Geometry check sheet. Reference: the model listing, model coordinates, mm. Coordinates: 2 decimals unless noted, no trailing zeros. Loops run counter-clockwise (first coordinate to the right, second up) from the corner with the lowest first, then second, coordinate; pieces in that order, holes last. Notation, with made-up numbers: (-35.5, 63) - (5.5, 63) arc R26 ccw to (5.5, 77) - close; hole circle Ø9 at (-36.75, 25). An arc over 180 degrees is marked (long way). One line per item, written item: value.
from build123d import *

# Parameters (mm, degrees)
SKETCH1_W           = 244
SKETCH1_H           = 158.15
BOSS_EXTRUDE1_DEPTH = 5
CUT_EXTRUDE1_DEPTH  = 10
SKETCH3_R           = 2.5
CUT_EXTRUDE2_DEPTH  = 10
SKETCH4_R           = 1
CUT_EXTRUDE3_DEPTH  = 10
SKETCH5_R           = 2
CUT_EXTRUDE4_DEPTH  = 10
CUT_EXTRUDE5_DEPTH  = 10


with BuildPart() as part:
    # Sketch1 → Boss-Extrude1 (new body)
    with BuildSketch(Plane.XY):
        with Locations((14.8, -10.925)):
            Rectangle(SKETCH1_W, SKETCH1_H)
    extrude(amount=BOSS_EXTRUDE1_DEPTH)

    # Sketch2 → Cut-Extrude1 (cut)
    with BuildSketch(Plane(origin=(0, 0, 0), x_dir=(-1, 0, 0), z_dir=(0, 0, -1))):
        Polygon((-136.8, 45.15), (-129.8, 45.15), (-129.8, 45.9), (-127.4, 45.9), (-127.4, 45.15), (-119.8, 45.15), (-119.8, 41.15), (-127.4, 41.15), (-127.4, 40.4), (-129.8, 40.4), (-129.8, 41.15), (-136.8, 41.15), align=None)
        Polygon((-129.8, -63), (-136.8, -63), (-136.8, -67), (-129.8, -67), (-129.8, -67.75), (-127.4, -67.75), (-127.4, -67), (-119.8, -67), (-119.8, -63), (-127.4, -63), (-127.4, -62.25), (-129.8, -62.25), align=None)
        Polygon((100.2, 41.15), (107.2, 41.15), (107.2, 45.15), (100.2, 45.15), (100.2, 45.9), (97.8, 45.9), (97.8, 45.15), (90.2, 45.15), (90.2, 41.15), (97.8, 41.15), (97.8, 40.4), (100.2, 40.4), align=None)
        Polygon((107.2, -67), (100.2, -67), (100.2, -67.75), (97.8, -67.75), (97.8, -67), (90.2, -67), (90.2, -63), (97.8, -63), (97.8, -62.25), (100.2, -62.25), (100.2, -63), (107.2, -63), align=None)
    extrude(amount=-CUT_EXTRUDE1_DEPTH, mode=Mode.SUBTRACT)

    # Sketch3 → Cut-Extrude2 (cut)
    with BuildSketch(Plane(origin=(0, 0, 0), x_dir=(-1, 0, 0), z_dir=(0, 0, -1))):
        with Locations((-124.8, -75.004567899)):
            Circle(SKETCH3_R)
        with Locations((-79.8, 48.15)):
            Circle(SKETCH3_R)
        with Locations((95.2, -75.004567899)):
            Circle(SKETCH3_R)
        with Locations((50.2, 48.15)):
            Circle(SKETCH3_R)
    extrude(amount=-CUT_EXTRUDE2_DEPTH, mode=Mode.SUBTRACT)

    # Sketch4 → Cut-Extrude3 (cut)
    with BuildSketch(Plane(origin=(0, 0, 0), x_dir=(-1, 0, 0), z_dir=(0, 0, -1))):
        with Locations((-38.8, 38.15)):
            Circle(SKETCH4_R)
        with Locations((1.2, 38.15)):
            Circle(SKETCH4_R)
        with Locations((-45.8, -32.925)):
            Circle(SKETCH4_R)
        with Locations((11.2, -32.925)):
            Circle(SKETCH4_R)
    extrude(amount=-CUT_EXTRUDE3_DEPTH, mode=Mode.SUBTRACT)

    # Sketch5 → Cut-Extrude4 (cut)
    with BuildSketch(Plane(origin=(0, 0, 0), x_dir=(-1, 0, 0), z_dir=(0, 0, -1))):
        with Locations((-64.634291995, 20.08216582)):
            Circle(SKETCH5_R)
        with Locations((37.798280732, 20.08216582)):
            Circle(SKETCH5_R)
        with Locations((37.798280732, -39.300167224)):
            Circle(SKETCH5_R)
        with Locations((-64.634291995, -39.300167224)):
            Circle(SKETCH5_R)
    extrude(amount=-CUT_EXTRUDE4_DEPTH, mode=Mode.SUBTRACT)

    # Sketch6 → Cut-Extrude5 (cut)
    with BuildSketch(Plane(origin=(0, 0, 0), x_dir=(-1, 0, 0), z_dir=(0, 0, -1))):
        with BuildLine():
            Line((-56.414434421, -72.751869016), (30.959965679, -72.751869016))
            ThreePointArc((30.959965679, -72.751869016), (39.799882323, -63.911952372), (30.959965679, -55.072035728))
            Line((30.959965679, -55.072035728), (-56.414434421, -55.072035728))
            ThreePointArc((-56.414434421, -55.072035728), (-65.254351065, -63.911952372), (-56.414434421, -72.751869016))
        make_face()
    extrude(amount=-CUT_EXTRUDE5_DEPTH, mode=Mode.SUBTRACT)


solid = part.part
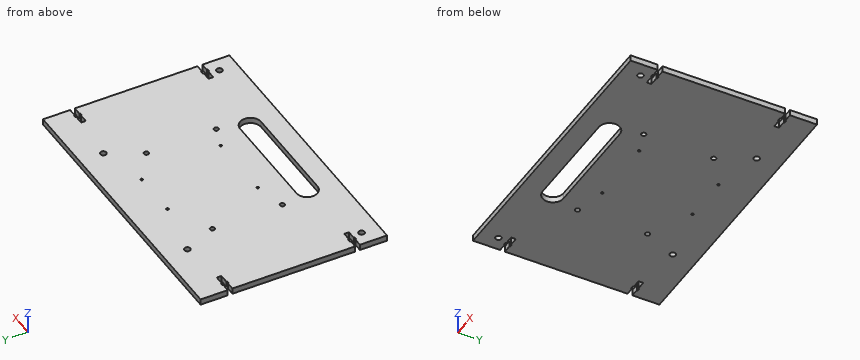
(1) Cross-section at A-A on x = 79.8. Record the cut outline in (y, z).
Reply:
outline: (-90, 0) - (45.65, 0) - (45.65, 5) - (-90, 5) - close; (50.65, 0) - (68.15, 0) - (68.15, 5) - (50.65, 5) - close
(2) Material ranges on probe 1 along Y at (x, z) = (-11.2, 3.35) (3 decimals); probe 2 along Y at (x, z) = (38.8, 2.3); probe 3 along Y at (x, z) = (-27, 4.65), recorded low to high. Write a range as from..to.
Reply:
probe 1: -90..-72.752, -55.072..-33.925, -31.925..68.15
probe 2: -90..-72.75, -55.07..37.15, 39.15..68.15
probe 3: -90..-72.75, -55.07..68.15
(3) Cross-section at C-C on z = 3.15. State how many separate pieces and enclosed holes the cut face has, and give its area (3 significant figures).
Reply:
separate pieces: 1
enclosed holes: 13
area: 36,400 mm2
(4) Go/stop test with a flat-tipped pin: pin 1 Ø3 at (x, y) = (124.8, -75) entering from -Z. Record where the tip stops, or that it passes through.
Reply:
pin 1: through
(5) Cross-section at B-B on x = -95.2. Record the cut outline in (y, z), and give its area (3 significant figures).
Reply:
outline: (-90, 0) - (-77.5, 0) - (-77.5, 5) - (-90, 5) - close; (-72.5, 0) - (-67, 0) - (-67, 5) - (-72.5, 5) - close; (-63, 0) - (41.15, 0) - (41.15, 5) - (-63, 5) - close; (45.15, 0) - (68.15, 0) - (68.15, 5) - (45.15, 5) - close
area: 726 mm2
